Here's how the part is built. I have some questions about the finished solid (model axes, mm). Face numbers are marked on the shaded views. Coordinates: 2 decimals unless noted, no trailing zeros. Order: outer loops, then holes, each group sorted by start corner. A loop starts at its lowest first (then second) coordinate and runs counter-clockwise, first axis right, second up. Notation, with made-up numbers: (65.25, 59.25) - (122.25, 59.25) arc R31 cw to (122.25, 91.25) - close; hole circle Ø7 at (63, -38.5). An arc over 180 degrees is marked (long way). Use one line per item in the form item = value. Start each with the question number.
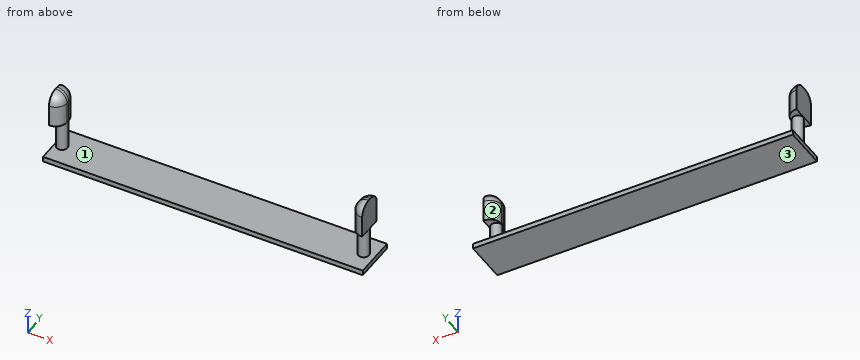
from build123d import *

# Parameters (mm, degrees)
F0_W     = 570.8396
F0_H     = 76.2
F1_DEPTH = 9.144
F2_R     = 9.651965
F3_DEPTH = 53.34
F4_W     = 20.748643
F4_H     = 45.828542
F5_DEPTH = 58.42
F6_R     = 20.32
F7_R     = 20.32


with BuildPart() as f1:
    # F0 (on Top) → F1 (new body)
    with BuildSketch(Plane.XY):
        with Locations((3.614875, 7.573666)):
            Rectangle(F0_W, F0_H)
    extrude(amount=F1_DEPTH)

    # F2 (on face) → F3 (join)
    with BuildSketch(Plane.XY.offset(9.144)):
        with Locations((-269.181566, 7.172334)):
            Circle(F2_R)
        with Locations((269.181566, 7.172334)):
            Circle(F2_R)
    extrude(amount=F3_DEPTH)

    # F4 (on face) → F5 (join)
    with BuildSketch(Plane.XY.offset(62.484)):
        with Locations((-269.181565, 7.172334)):
            Rectangle(F4_W, F4_H)
        with Locations((269.181565, 7.172334)):
            Rectangle(F4_W, F4_H)
    extrude(amount=F5_DEPTH)

    # F6
    f6_edges = [f1.edges().sort_by_distance(p)[0] for p in [
        (-269.181566, -15.741937, 120.904),
        (-258.807244, 7.172334, 120.904),
        (-269.181566, 30.086605, 120.904),
        (-258.807244, -15.741937, 91.694),
        (-258.807244, 30.086605, 91.694),
    ]]
    fillet(f6_edges, radius=F6_R)

    # F7
    f7_edges = [f1.edges().sort_by_distance(p)[0] for p in [
        (258.807244, 7.172334, 120.904),
        (258.807244, 30.086605, 91.694),
        (258.807244, -15.741937, 91.694),
        (269.181566, -15.741937, 120.904),
        (269.181566, 30.086605, 120.904),
    ]]
    fillet(f7_edges, radius=F7_R)


solid = f1.part
1) For pin 1 (13.5 mm diameter, centred on y = 17.5, z = 105.5, fed in from +X); pin 2 (0.5 mm diameter, centred on x = -279.5, z = 83, fed in from -Y); pin 3 (10 mm diameter, centred on x = -153.5, y = 32, fed in from +Z), each with a flat end and sliding along its axis, tell me the tip position at first contact or that it passes through.
2) Suppose I cut it at B-B, the plane x = -242. List the corners of the cut face in (y, z) for me.
3) I need wall thicknesses on probe 1 along X at (y, z) = (4.5, 72.5); probe 2 along Z at (x, y) = (2, 15); probe 3 along X at (y, z) = (4, 57). Which ranges of each line are inside material? Lowest first, please. Write a range as [from, to].
4) Suppose I cut it at A-A, the plane z = 95. List the corners of the cut face in (x, y) for me.
5) Suppose I cut it at C-C, the plane y = 38.5. List the corners of the cut face in (x, z) for me.
6) If we mould it in two halves opening along X, with no side actions, what happens to the marked faces 1, 2 and 3? For each: pulls with the +X half, pulls with the -X half, needs draft (parallel to the pull), parting line crosses it, or undercut.
7) Suppose I cut it at D-D, the plane z = 49. List the corners of the cut face in (x, y) for me, then the cut area to 3 significant figures.
From the geometry:
q1.pin_1 = 279.56
q1.pin_2 = -15.74
q1.pin_3 = 9.14
q2.outline = (-30.53, 0) - (45.67, 0) - (45.67, 9.14) - (-30.53, 9.14) - close
q3.probe_1 = [-279.56, -258.81], [258.81, 279.56]
q3.probe_2 = [0, 9.14]
q3.probe_3 = [-278.3, -260.07], [260.07, 278.3]
q4.outline = (-279.56, -15.74) - (-279.13, -15.74) arc R20.32 ccw to (-258.81, 4.58) - (-258.81, 9.77) arc R20.32 ccw to (-279.13, 30.09) - (-279.56, 30.09) - close; (258.81, 4.58) arc R20.32 ccw to (279.13, -15.74) - (279.56, -15.74) - (279.56, 30.09) - (279.13, 30.09) arc R20.32 ccw to (258.81, 9.77) - close
q5.outline = (-281.8, 0) - (289.03, 0) - (289.03, 9.14) - (-281.8, 9.14) - close
q6.face_1 = undercut
q6.face_2 = undercut
q6.face_3 = needs draft
q7.outline = circle Ø19.3 at (-269.18, 7.17); circle Ø19.3 at (269.18, 7.17)
q7.area = 585 mm2
